For this review, use the dimensioned drawing (mm, ordinates from the lowest corner) and the shaded views. Coordinates: 2 decimals unless noted, no trailing zeros. Order: outer loops, then holes, each group sorted by start corner. A loop starts at its lowest first (then second) coordinate and runs counter-clockwise, first axis right, second up. Notation, with made-up numbers: M 46,39 L 71,39 A30 cw 71,74 Z; hole C 55,-27.5 d2. An arc over 180 degrees is marked long. Use one line per item in the form item = value. Start each with the question number.
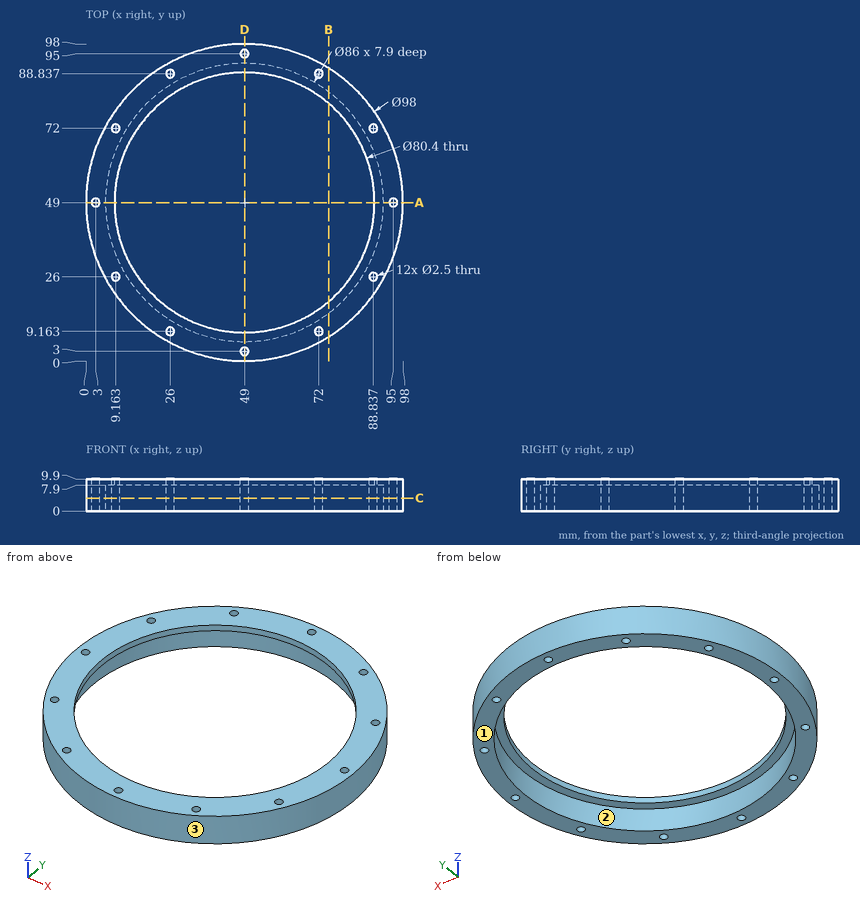
1. Consider section C-C, the plane z = 4. Give the number of separate pieces and of enclosed holes in the cut face, plus the area to 3 significant figures.
2. Consider section A-A, the plane y = 49. Write out the cut boundary in (x, z), plus the area to 3 significant figures.
3. The part is to be moulded in two halves that separate along X. For the marked faces 1, 2 and 3, say which applies: pulls with the +X half, pulls with the -X half, needs draft (parallel to the pull), parting line crosses it, or undercut.
4. For pin 1 Ø3 at (x, y) = (9.16, 26) entering from -Z; pin 2 Ø5 at (y, z) = (18.5, 6) entering from +X; pin 3 Ø5 at (y, z) = (57.5, 2) entering from +X, all flat-tipped, find the tip position at first contact; note any pin that passes through.
5. Consider section B-B, the plane x = 75. Write out the cut boundary in (y, z).
6. To check wall thickness, follow line 1 (X direction, y = 72, z = 2.5); line 2 (Y direction, x = 57, z = 4.25); line 3 (Y direction, x = 69, z = 3.25). State the ranges of each line that lie inside material, in increasing order.
Answers follow:
q1.separate_pieces = 1
q1.enclosed_holes = 13
q1.area = 1,680 mm²
q2.outline = M 0,0 L 1.75,0 L 1.75,9.9 L 0,9.9 Z; M 4.25,0 L 6,0 L 6,7.9 L 8.8,7.9 L 8.8,9.9 L 4.25,9.9 Z; M 89.2,7.9 L 92,7.9 L 92,0 L 93.75,0 L 93.75,9.9 L 89.2,9.9 Z; M 96.25,0 L 98,0 L 98,9.9 L 96.25,9.9 Z
q2.area = 80.5 mm²
q3.face_1 = needs draft
q3.face_2 = undercut
q3.face_3 = parting line crosses it
q4.pin_1 = 0
q4.pin_2 = 89.21
q4.pin_3 = 97.63
q5.outline = M 7.47,0 L 14.75,0 L 14.75,7.9 L 18.34,7.9 L 18.34,9.9 L 7.47,9.9 Z; M 79.66,7.9 L 83.25,7.9 L 83.25,0 L 90.53,0 L 90.53,9.9 L 79.66,9.9 Z
q6.line_1 = 5.73 to 7.91, 10.41 to 12.67, 85.33 to 87.59, 90.09 to 92.27
q6.line_2 = 0.66 to 6.75, 91.25 to 97.34
q6.line_3 = 4.27 to 10.93, 87.07 to 93.73
